Here's the drawing with two shaded views (mm, measured from the low corner). I have some questions. A direction names the side the tool comes from. Give positions to 0.01 mm unless a question says otherwise; leave off trailing zeros. Order: outer loops, then holes, each group sorted by start corner. A loop starts at its lowest first (then second) coordinate and runs counter-clockwise, first axis right, second up. Notation, with made-up numbers: (21, 71) - (72, 71) arc R11 cw to (72, 85) - close; hole circle Ø1 at (61.25, -30.75). An arc over 180 degrees is marked (long way). Use one line per item in the form item = value. Start each with the question number.
1) Suppose I cut it at B-B, the plane x = 43. Write out the boundary of the cut face in (y, z).
2) Which directions (+Z, -Z, +X, -X, +Y, -Y) give clear straight access to the entire face, cutting with the end or side of a thin tool? Please do the marked faces 1, 2 and 3.
3) Suppose I cut it at C-C, the plane y = 18. Write out the boundary of the cut face in (x, z), and give its area (4 significant figures).
4) For pin 1 (9 mm diameter, centred on x = 20.5, y = 86, fed in from -Z); pin 2 (12 mm diameter, centred on y = 22, z = 37.5, fed in from +X); pin 3 (8 mm diameter, centred on x = 16, y = 29, fed in from -Z), each with a flat end and sliding along its axis, tell me the tip position at first contact or that it passes through.
5) Please list where these lines run through material, in increasing order: probe 1 along Z at (x, y) = (29, 71.5); probe 2 along X at (y, z) = (84.5, 28).
6) Suppose I cut it at A-A, the plane z = 17.5. Write out the boundary of the cut face in (x, y), and give its area (3 significant figures).
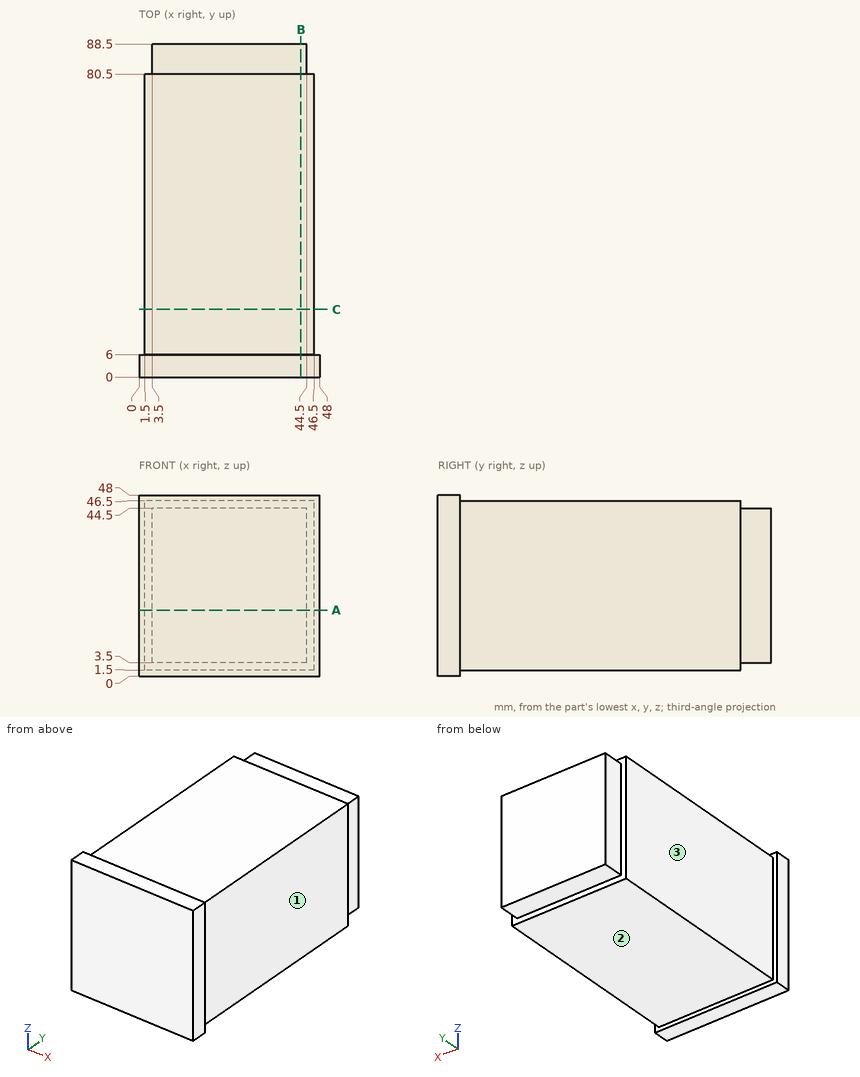
Result sheet:
q1.outline = (0, 0) - (6, 0) - (6, 1.5) - (80.5, 1.5) - (80.5, 3.5) - (88.5, 3.5) - (88.5, 44.5) - (80.5, 44.5) - (80.5, 46.5) - (6, 46.5) - (6, 48) - (0, 48) - close
q2.face_1 = +Z, -Z, +X, +Y
q2.face_2 = -Z, +X, -X, +Y
q2.face_3 = +Z, -Z, -X, +Y
q3.outline = (1.5, 1.5) - (46.5, 1.5) - (46.5, 46.5) - (1.5, 46.5) - close
q3.area = 2,025 mm²
q4.pin_1 = 3.5
q4.pin_2 = 46.5
q4.pin_3 = 1.5
q5.probe_1 = 1.5 to 46.5
q5.probe_2 = 3.5 to 44.5
q6.outline = (0, 0) - (48, 0) - (48, 6) - (46.5, 6) - (46.5, 80.5) - (44.5, 80.5) - (44.5, 88.5) - (3.5, 88.5) - (3.5, 80.5) - (1.5, 80.5) - (1.5, 6) - (0, 6) - close
q6.area = 3,970 mm²
